```python
from build123d import *

# Parameters (mm, degrees)
BOSS_EXTRUDE1_DEPTH = 203.2
SHELL1_T            = -3.048
FILLET1_R           = 2.54
SKETCH2_R           = 3.175
CUT_EXTRUDE1_DEPTH  = 203.2


with BuildPart() as part:
    # Sketch1 → Boss-Extrude1 (new body)
    with BuildSketch(Plane.XY):
        with BuildLine():
            Line((-11.300558575, 134.809128263), (34.419441425, 134.809128263))
            ThreePointArc((34.419441425, 134.809128263), (36.215492649, 134.065179487), (36.959441425, 132.269128263))
            Line((36.959441425, 132.269128263), (36.959441425, -15.050871737))
            ThreePointArc((36.959441425, -15.050871737), (36.215492649, -16.846922961), (34.419441425, -17.590871737))
            Line((34.419441425, -17.590871737), (-11.300558575, -17.590871737))
            ThreePointArc((-11.300558575, -17.590871737), (-13.096609799, -16.846922961), (-13.840558575, -15.050871737))
            Line((-13.840558575, -15.050871737), (-13.840558575, 132.269128263))
            ThreePointArc((-13.840558575, 132.269128263), (-13.096609799, 134.065179487), (-11.300558575, 134.809128263))
        make_face()
    extrude(amount=BOSS_EXTRUDE1_DEPTH)

    # Shell1
    shell1_openings = [part.faces().sort_by_distance(p)[0] for p in [
        (11.559441425, 58.609128263, 203.2),
        (11.559441425, 58.609128263, 0),
    ]]
    offset(amount=SHELL1_T, openings=shell1_openings, kind=Kind.INTERSECTION)

    # Fillet1
    fillet1_edges = [part.edges().sort_by_distance(p)[0] for p in [
        (33.911441425, -14.542871737, 101.6),
        (33.911441425, 131.761128263, 101.6),
        (-10.792558575, 131.761128263, 101.6),
        (-10.792558575, -14.542871737, 101.6),
    ]]
    fillet(fillet1_edges, radius=FILLET1_R)

    # Sketch2 → Cut-Extrude1 (cut)
    with BuildSketch(Plane(origin=(36.959441425, 0, 0), x_dir=(0, 0, -1), z_dir=(1, 0, 0))):
        with Locations(Location((-52.07, 58.609128263, 0), (0, 0, 90))):
            Circle(SKETCH2_R)
        with Locations(Location((-85.09, 58.609128263, 0), (0, 0, 90))):
            Circle(SKETCH2_R)
        with Locations(Location((-118.11, 58.609128263, 0), (0, 0, 90))):
            Circle(SKETCH2_R)
        with Locations(Location((-151.13, 58.609128263, 0), (0, 0, 90))):
            Circle(SKETCH2_R)
        with Locations(Location((-184.15, 58.609128263, 0), (0, 0, 90))):
            Circle(SKETCH2_R)
        with Locations(Location((-19.05, 58.609128263, 0), (0, 0, 90))):
            Circle(SKETCH2_R)
    extrude(amount=-CUT_EXTRUDE1_DEPTH, mode=Mode.SUBTRACT)


solid = part.part
```
Here's how the part is built. I have some questions about the finished solid (model axes, mm). A direction names the side the tool comes from. Give positions to 0.01 mm unless a question says otherwise; leave off trailing zeros. Write each loop counter-clockwise with the first axis right and the second up, starting at its lowest first coordinate (ties: lowest second). Pieces come first, ordered by that corner, then holes. Notation, with made-up numbers: M 82,-18.75 L 127,-18.75 A33 ccw 127,10.25 Z; hole C 31,78 d3. An arc over 180 degrees is marked long. Put each result on its own line as item: value. Start each with the question number.
Item 1: On a 3-axis mill with a long thin cutter (end or side, diameter ignored), from which of +Z, -Z, +X, -X, +Y, -Y can I reach the whole of each face in a straight line? I mean faces 4 (the flat face through (-10.793, 58, 100)), 5 (the cylindrical face through (-12.295, 56.269, 54.216)). Say none if no direction works.
Item 2: If we section it at C-C, the plane x = 11: Write out the boundary of the cut face in (y, z), then the cut area to 3 significant figures.
Item 3: If we section it at A-A, the plane z = 184.15: Write out the boundary of the cut face in (x, y), then the cut area to 3 significant figures.
Item 4: Will this pin go through, and if not, where does the flat tip stop? pin 1 (5.5 mm diameter, centred on y = 58.61, z = 85.09, fed in from -X).
Item 5: If we section it at D-D, the plane z = 66: Write out the boundary of the cut face in (x, y), then the cut area to 3 significant figures.
Item 6: I need wall thicknesses on L1, parallel to Y at x = 34, z = 184; L2, parallel to X at y = -2.5, z = 31.5; L3, parallel to Y at x = -5.5, z = 116. Which ranges of each line are inside material? Lowest first, please. Write a range as from..to.
Item 7: If we section it at B-B, the plane y = 21.5: Write out the boundary of the cut face in (x, z).
Item 8: Thinking about a two-plate mould opening in Z: for faces 1 (the cylindrical face through (35.46, 57.92, 15.95)), 2 (the flat face through (34.3, 70.3, 0)), 3 (the flat face through (11, 131.761, 100)), which applies, +Z half, -Z half, draft (parallel to the pull), parting line (faces both ways), or undercut?
Values:
1. face 4: +Z, -Z
1. face 5: +X, -X
2. outline: M -17.59,0 L -14.54,0 L -14.54,203.2 L -17.59,203.2 Z; M 131.76,0 L 134.81,0 L 134.81,203.2 L 131.76,203.2 Z
2. area: 1,240 mm²
3. outline: M -13.84,-15.05 A2.54 ccw -11.3,-17.59 L 34.42,-17.59 A2.54 ccw 36.96,-15.05 L 36.96,55.43 L 33.91,55.43 L 33.91,-12 A2.54 cw 31.37,-14.54 L -8.25,-14.54 A2.54 cw -10.79,-12 L -10.79,55.43 L -13.84,55.43 Z; M -13.84,61.78 L -10.79,61.78 L -10.79,129.22 A2.54 cw -8.25,131.76 L 31.37,131.76 A2.54 cw 33.91,129.22 L 33.91,61.78 L 36.96,61.78 L 36.96,132.27 A2.54 ccw 34.42,134.81 L -11.3,134.81 A2.54 ccw -13.84,132.27 Z
3. area: 1,160 mm²
4. pin 1: through
5. outline: M -13.84,-15.05 A2.54 ccw -11.3,-17.59 L 34.42,-17.59 A2.54 ccw 36.96,-15.05 L 36.96,132.27 A2.54 ccw 34.42,134.81 L -11.3,134.81 A2.54 ccw -13.84,132.27 Z; hole M -10.79,-12 A2.54 ccw -8.25,-14.54 L 31.37,-14.54 A2.54 ccw 33.91,-12 L 33.91,129.22 A2.54 ccw 31.37,131.76 L -8.25,131.76 A2.54 ccw -10.79,129.22 Z
5. area: 1,200 mm²
6. L1: -17.59..55.44, 61.78..134.81
6. L2: -13.84..-10.79, 33.91..36.96
6. L3: -17.59..-14.54, 131.76..134.81
7. outline: M -13.84,0 L -10.79,0 L -10.79,203.2 L -13.84,203.2 Z; M 33.91,0 L 36.96,0 L 36.96,203.2 L 33.91,203.2 Z
8. face 1: undercut
8. face 2: -Z half
8. face 3: draft
